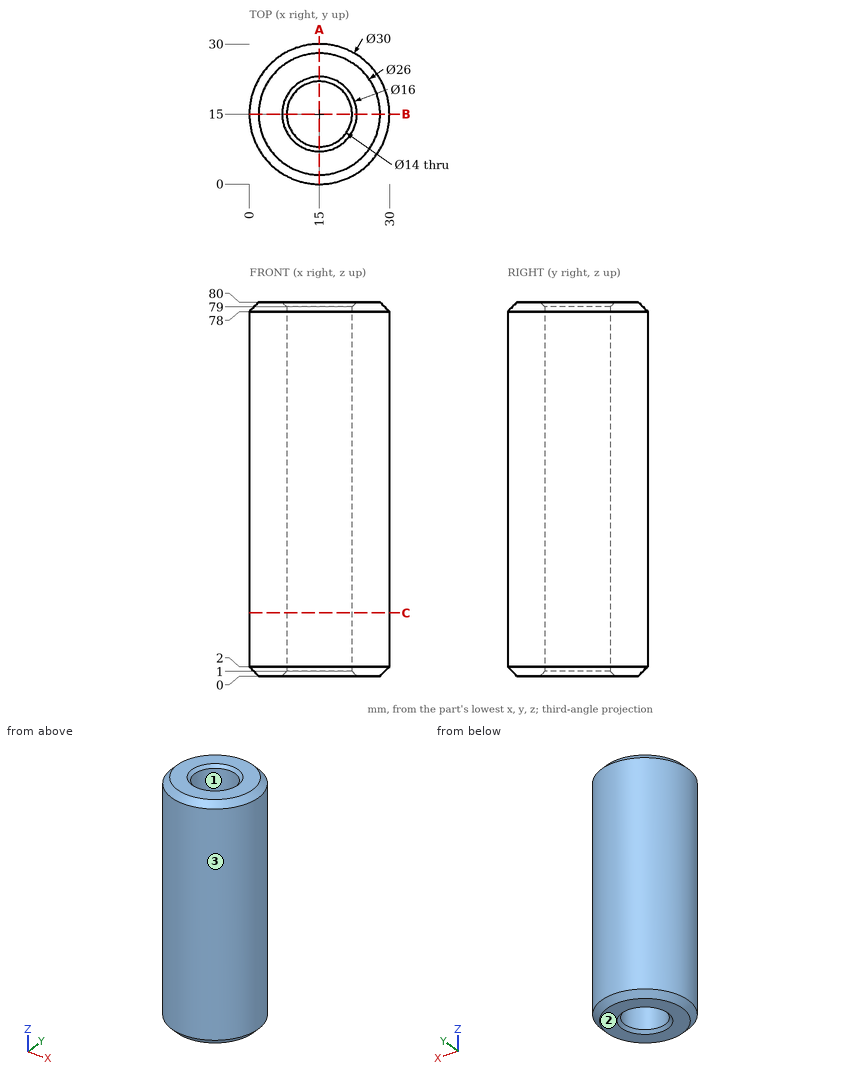
Geometry: see drawing. Coordinates: mm, zero at the bounding-box minimum. Give positions to 0.01 mm unless a question says otherwise; leave off trailing zeros. Loops run counter-clockwise (first coordinate to the right, second up) from the corner with the lowest first, then second, coordinate; pieces in that order, holes last. Notation, with made-up numbers: (4.5, 39.5) - (17.5, 39.5) arc R19 cw to (17.5, 52.5) - close; hole circle Ø4 at (13.25, 10). An arc over 180 degrees is marked (long way). Use CSV: the item, a comma, the result in double quotes.
1) Line query: line 1 (Y direction, x = 15, z = 57); line 2 (Y direction, x = 11, z = 45); line 3 (Z direction, x = 24, y = 4.5). Output: solid intervals per line, ascending.
Worked out:
line 1,"y = 0 to 8, 22 to 30"
line 2,"y = 0.54 to 9.26, 20.74 to 29.46"
line 3,"z = 0.83 to 79.17"
2) Cut plane C-C (z = 13.5). Output: boundary loops of the cut face in (x, y).
Worked out:
outline,"circle Ø30 at (15, 15); hole circle Ø14 at (15, 15)"
3) Cut plane A-A (x = 15). Output: boundary loops of the cut face in (y, z).
Worked out:
outline,"(0, 2) - (2, 0) - (7, 0) - (8, 1) - (8, 79) - (7, 80) - (2, 80) - (0, 78) - close; (22, 1) - (23, 0) - (28, 0) - (30, 2) - (30, 78) - (28, 80) - (23, 80) - (22, 79) - close"
4) Mould query, pull axis Y, two halves, no side actions, for the marked faces 1, 2 and 3. Classes: +Y half, -Y half, draft (parallel to the pull), parting line (faces both ways), or undercut.
Worked out:
face 1,"undercut"
face 2,"draft"
face 3,"parting line"
5) Pin query (flat end, axial travel): P1, Ø6, axis at y = 13.5, z = 48.5, coming from the +X side; P2, Ø1, axis at y = 17, z = 31.5, coming from the -X side; P3, Ø6, axis at y = 21, z = 36.5, coming from the -X side; P4, Ø2, axis at x = 23.5, z = 19, coming from the +Y side. Return the tip coordinate at first contact, or that it passes through.
Worked out:
P1,"stops at x = 30"
P2,"stops at x = 0.08"
P3,"stops at x = 0.3"
P4,"stops at y = 27.99"
